Input: part model. Units: mm. Frame: model coordinates. Coordinates: 2 decimals unless noted, no trailing zeros. Write each loop counter-clockwise with the first axis right and the second up, starting at its lowest first coordinate (ties: lowest second). Pieces come first, ordered by that corner, then holes. Notation, with made-up numbers: (-38, 12.25) - (15, 12.25) arc R6 ccw to (15, 19.25) - close; hole circle Ø11 at (-19.5, 77). An arc over 180 degrees is marked (long way). Use a Markdown table: item, result. Add a question column.
Q1. Section query A-A (y = -582.5). Return the cut outline in (x, z).
Q2. Section query B-B (x = -111). Return the cut outline in (y, z).
Q3. Material intervals for probe 1 along Z at (x, y) = (112, 534), sorted ascending. Write a range as from..to.
Q4. Pin query (flat end, axial travel): P1, Ø0.7, axis at y = 36, z = 11, coming from the +X side; P2, Ø5, axis at x = -116.5, y = 585.5, coming from the +Z side; P3, Ø1.9, axis at x = 247.5, z = 9, coming from the +Y side; P4, Ø6, axis at x = -185.5, z = 10.5, coming from the -Y side. Return the tip coordinate at first contact, or that it passes through.
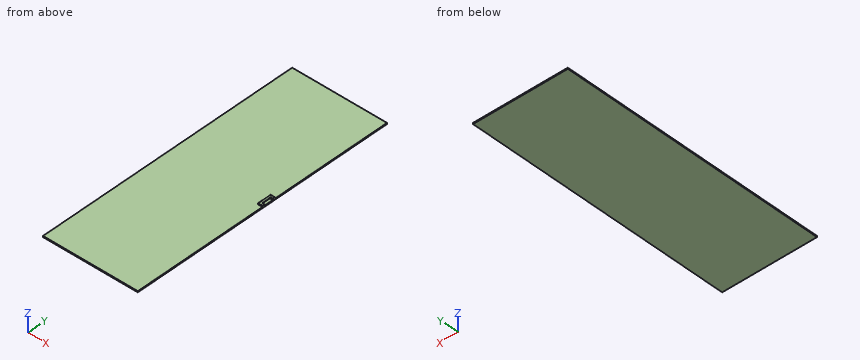
from build123d import *

# Parameters (mm, degrees)
SKETCH1_W           = 520.7
SKETCH1_H           = 1473.2
BOSS_EXTRUDE1_DEPTH = 6.35
BOSS_EXTRUDE2_DEPTH = 6.35
SKETCH2_4_W         = 10.0763546
SKETCH2_4_H         = 50.817669104
CUT_EXTRUDE1_DEPTH  = 3.175
SKETCH4_W           = 4.7625
SKETCH4_H           = 50.817669104
CUT_EXTRUDE2_DEPTH  = 6.35
FILLET1_R           = 2.54
FILLET2_R           = 2.54


with BuildPart() as part:
    # Sketch1 → Boss-Extrude1 (new body)
    with BuildSketch(Plane.XY):
        Rectangle(SKETCH1_W, SKETCH1_H)
    extrude(amount=BOSS_EXTRUDE1_DEPTH)

    # Sketch2 → Boss-Extrude2 (add)
    with BuildSketch(Plane.XY.offset(6.35)):
        Polygon((234.95, 0), (260.35, 0), (260.35, 12.620459264), (257.7263546, 12.620459264), (247.65, 12.620459264), (247.65, 63.438128368), (257.7263546, 63.438128368), (260.35, 63.438128368), (260.35, 76.2), (234.95, 76.2), align=None)
    extrude(amount=BOSS_EXTRUDE2_DEPTH)

    # Sketch2<4> → Cut-Extrude1 (cut)
    with BuildSketch(Plane.XY.offset(6.35)):
        with Locations((252.6881773, 38.029293816)):
            Rectangle(SKETCH2_4_W, SKETCH2_4_H)
    extrude(amount=-CUT_EXTRUDE1_DEPTH, mode=Mode.SUBTRACT)

    # Sketch4 → Cut-Extrude2 (cut)
    with BuildSketch(Plane(origin=(247.65, 0, 0), x_dir=(0, 0, -1), z_dir=(1, 0, 0))):
        with Locations((-5.55625, 38.029293816)):
            Rectangle(SKETCH4_W, SKETCH4_H)
    extrude(amount=-CUT_EXTRUDE2_DEPTH, mode=Mode.SUBTRACT)

    # Fillet1
    fillet1_edges = [part.edges().sort_by_distance(p)[0] for p in [
        (247.65, 38.029293816, 7.9375),
    ]]
    fillet(fillet1_edges, radius=FILLET1_R)

    # Fillet2
    fillet2_edges = [part.edges().sort_by_distance(p)[0] for p in [
        (234.95, 38.1, 12.7),
        (247.65, 0, 12.7),
        (260.35, 69.819064184, 12.7),
        (247.65, 76.2, 12.7),
        (260.35, 6.310229632, 12.7),
    ]]
    fillet(fillet2_edges, radius=FILLET2_R)


solid = part.part
Values follow:
| question | item | result |
|---|---|---|
| 1 | outline | (-260.35, 0) - (260.35, 0) - (260.35, 6.35) - (-260.35, 6.35) - close |
| 2 | outline | (-736.6, 0) - (736.6, 0) - (736.6, 6.35) - (-736.6, 6.35) - close |
| 3 | probe 1 | 0..6.35 |
| 4 | P1 | x = 247.65 |
| 4 | P2 | z = 6.35 |
| 4 | P3 | y = 76.2 |
| 4 | P4 | through |
